Autodesk Inventor part; units mm, degrees
ref_plane "YZ Plane" through (0, 0, 0) normal (1, 0, 0) x (0, 1, 0)
ref_plane "XZ Plane" through (0, 0, 0) normal (0, 1, 0) x (-1, 0, 0)
ref_plane "XY Plane" through (0, 0, 0) normal (0, 0, 1) x (1, 0, 0)
sketch "Esquisse1" plane through (0, 0, 0) normal (1, 0, 0) x (0, 1, 0)
  circle A0 centre (0, 0) radius 1.5
  dimension "d0" = 3
extrude "Extrusion1" add sketch "Esquisse1" along normal mid plane 15
chamfer "Chanfrein2" distance 3 angle 15 1 edges at (7.5, -1.5, 0) measured on face at (5, 1.4951, -0.1207)
chamfer "Chanfrein3" distance 3 angle 15 1 edges at (-7.5, -1.5, 0) measured on face at (-5, 1.4951, -0.1207)
properties part number "goupille"
Could you check a few things on this model? Use its own coordinates, in mm. Give positions to 0.01 mm unless a question says otherwise; leave off trailing zeros. Loops run counter-clockwise (first coordinate to the right, second up) from the corner with the lowest first, then second, coordinate; pieces in that order, holes last. Notation, with made-up numbers: (2, -23.75) -> (60, -23.75) arc R25 ccw to (60, -3.75) -> close; hole circle Ø10 at (16, 63.25). An arc over 180 degrees is marked (long way). Return JSON: item names as keys, results as strings.
Item 1: If we section it at C-C on x = -3.5: List the corners of the cut face in (y, z) for me.
Geometry results:
{"outline": "circle Ø3 at (0, 0)"}
Item 2: If we section it at D-D on x = -5.5: List the corners of the cut face in (y, z) for me, plus the area to 3 significant figures.
Geometry results:
{"outline": "circle Ø2.46 at (0, 0)", "area": "4.77 mm²"}
Item 3: If we section it at A-A on z = 0: List the corners of the cut face in (x, y) for me.
Geometry results:
{"outline": "(-7.5, -0.7) -> (-4.5, -1.5) -> (4.5, -1.5) -> (7.5, -0.7) -> (7.5, 0.7) -> (4.5, 1.5) -> (-4.5, 1.5) -> (-7.5, 0.7) -> close"}
Item 4: I need wall thicknesses on L1, parallel to Z at x = 2.25, y = 1.1; L2, parallel to Y at x = 0.25, z = -0.1; L3, parallel to Z at x = 0.75, y = 0.15. Which ranges of each line are inside material? Lowest first, please. Write a range as from..to.
Geometry results:
{"L1": "z = -1.02..1.02", "L2": "y = -1.5..1.5", "L3": "z = -1.49..1.49"}
Item 5: I'm going to push a flat-ended pin straight in: pin 1 (1.5 mm diameter, centred on x = 5.5, z = 1, fed in from +Y). Where does the tip first touch, or does it pass through?
Geometry results:
{"pin 1": "stops at y = 1.29"}
